Model file for the job. Use its own axes, mm. A direction names the side the tool comes from. Coordinates: 2 decimals unless noted, no trailing zeros. Write each loop counter-clockwise with the first axis right and the second up, starting at its lowest first coordinate (ties: lowest second). Pieces come first, ordered by that corner, then holes. Notation, with made-up numbers: M 43,73.5 L 64,73.5 A15 cw 64,88.5 Z; hole C 38.5,-22 d5. An arc over 180 degrees is marked long. Use CSV: the item, a comma, the result in double quotes. Start each with the question number.
from build123d import *

# Parameters (mm, degrees)
F0_W     = 165.1
F0_H     = 38.1
F1_DEPTH = 88.9
F2_W     = 50.8
F2_H     = 12.7
F3_DEPTH = 165.1
F4_W     = 165.1
F4_H     = 19.05
F5_DEPTH = 12.7
F6_DEPTH = 12.7
F7_R     = 12.7
F8_DEPTH = 25.4
F9_DEPTH = 25.4


with BuildPart() as f1:
    # F0 (on Front) → F1 (new body)
    with BuildSketch(Plane.XZ):
        with Locations((82.55, 19.05)):
            Rectangle(F0_W, F0_H)
    extrude(amount=F1_DEPTH)

    # F2 (on face) → F3 (cut)
    with BuildSketch(Plane.YZ.offset(165.1)):
        with Locations((-44.45, 6.35)):
            Rectangle(F2_W, F2_H)
    extrude(amount=-F3_DEPTH, mode=Mode.SUBTRACT)

    # F4 (on face) → F5 (cut)
    with BuildSketch(Plane.XY.offset(38.1)):
        with Locations((82.55, -79.375)):
            Rectangle(F4_W, F4_H)
    extrude(amount=-F5_DEPTH, mode=Mode.SUBTRACT)

    # F4 (on face) → F6 (cut)
    with BuildSketch(Plane.XY.offset(38.1)):
        with Locations((82.55, -9.525)):
            Rectangle(F4_W, F4_H)
    extrude(amount=-F6_DEPTH, mode=Mode.SUBTRACT)

    # F7 (on face) → F8 (cut, through all)
    with BuildSketch(Plane.XY.offset(38.1)):
        with Locations((130.175, -44.45)):
            Circle(F7_R)
    extrude(amount=-F8_DEPTH, mode=Mode.SUBTRACT)

    # F7 (on face) → F9 (cut, through all)
    with BuildSketch(Plane.XY.offset(38.1)):
        with Locations((34.925, -44.45)):
            Circle(F7_R)
    extrude(amount=-F9_DEPTH, mode=Mode.SUBTRACT)


solid = f1.part
1) Two-plate mould, pull along X, no slides. Class faces 1 (the face through (165.1, -44, 19)), 2 (the face through (25.56, -35.87, 25.58)), 3 (the face through (84, -45, 12.7)): pulls with the +X half, pulls with the -X half, needs draft (parallel to the pull), parting line crosses it, or undercut.
2) Tool access for faces 4 (the face through (81, 0, 13)), 5 (the face through (84, -69.85, 6)), 6 (the face through (81, -9, 25.4)), 7 (the face through (81, -69.85, 32)): list every direction of +Z, -Z, +X, -X, +Y, -Y with a clear straight run to the whole face (end or side of a thin tool).
3) Drop flat-ended pins along their axis: P1, Ø3, axis at x = 28, y = -72, coming from the +Z side; P2, Ø1.5, axis at x = 117, z = 31, coming from the +Y side; P3, Ø6, axis at x = 97.5, y = -34, coming from the -Z side. Give the stop position or say it passes through.
4) Band-saw the part on A-A on y = -44.45. List the corners of the cut face in (x, z) (3 decimals), then the cut area to 3 significant figures.
5) Band-saw the part on C-C on z = 34.5. List the corners of the cut face in (x, y) (3 decimals).
6) Band-saw the part on D-D on x = 122. List the corners of the cut face in (y, z).
7) Wall check: L1, parallel to X at y = -44, z = 32; L2, parallel to Y at x = 112, z = 7; L3, parallel to X at y = -47, z = 13.5. Give the ranges that are in metal, low to high. Write a range as [from, to].
8) Band-saw the part on B-B on x = 17.5. List the corners of the cut face in (y, z), then the cut area to 3 significant figures.
Findings below:
1,face 1,"pulls with the +X half"
1,face 2,"undercut"
1,face 3,"needs draft"
2,face 4,"+Z, -Z, +X, -X, +Y"
2,face 5,"-Z, +X, -X"
2,face 6,"+Z, +X, -X, +Y"
2,face 7,"+Z, +X, -X, -Y"
3,P1,"stops at z = 25.4"
3,P2,"stops at y = -19.05"
3,P3,"stops at z = 12.7"
4,outline,"M 0,12.7 L 22.225,12.7 L 22.225,38.1 L 0,38.1 Z; M 47.625,12.7 L 117.475,12.7 L 117.475,38.1 L 47.625,38.1 Z; M 142.875,12.7 L 165.1,12.7 L 165.1,38.1 L 142.875,38.1 Z"
4,area,"2,900 mm2"
5,outline,"M 0,-69.85 L 165.1,-69.85 L 165.1,-19.05 L 0,-19.05 Z; hole C 34.925,-44.45 d25.4; hole C 130.175,-44.45 d25.4"
6,outline,"M -88.9,0 L -69.85,0 L -69.85,12.7 L -54.17,12.7 L -54.17,38.1 L -69.85,38.1 L -69.85,25.4 L -88.9,25.4 Z; M -34.73,12.7 L -19.05,12.7 L -19.05,0 L 0,0 L 0,25.4 L -19.05,25.4 L -19.05,38.1 L -34.73,38.1 Z"
7,L1,"x = [0, 22.23], [47.62, 117.48], [142.87, 165.1]"
7,L2,"y = [-88.9, -69.85], [-19.05, 0]"
7,L3,"x = [0, 22.48], [47.37, 117.73], [142.62, 165.1]"
8,outline,"M -88.9,0 L -69.85,0 L -69.85,12.7 L -19.05,12.7 L -19.05,0 L 0,0 L 0,25.4 L -19.05,25.4 L -19.05,38.1 L -69.85,38.1 L -69.85,25.4 L -88.9,25.4 Z"
8,area,"2,260 mm2"
